Check sheet for the modelled part. Datum: model origin and axes. Units: mm. Round coordinates to 2 decimals unless told otherwise and drop trailing zeros. Order: outer loops, then holes, each group sorted by start corner. A loop starts at its lowest first (then second) coordinate and runs counter-clockwise, first axis right, second up. Notation, with made-up numbers: (87, 1) -> (108, 1) arc R14 ccw to (108, 27) -> close; hole circle Ø6 at (-30, 72.25). An arc over 180 degrees is marked (long way). Answer in a Markdown table with one row per item.
```python
from build123d import *

# Parameters (mm, degrees)
BOSS_EXTRUDE1_DEPTH = 250
BOSS_EXTRUDE3_START = -17.1
SKETCH3_W           = 10
SKETCH3_H           = 10
SKETCH3_R           = 1.75
BOSS_EXTRUDE3_DEPTH = 7
FILLET1_R           = 5
SKETCH5_R           = 1.5
CUT_EXTRUDE1_DEPTH  = 7
SKETCH6_W           = 20
SKETCH6_H           = 5
BOSS_EXTRUDE4_DEPTH = 7
SKETCH2_R           = 8.1
BOSS_EXTRUDE5_DEPTH = 5
BOSS_EXTRUDE6_START = -25
SKETCH2_3_R         = 8.1
BOSS_EXTRUDE6_DEPTH = 5
SKETCH7_R           = 1.5
CUT_EXTRUDE2_DEPTH  = 254.574446662


with BuildPart() as part:
    # Sketch1 → Boss-Extrude1 (new body)
    with BuildSketch(Plane.XY):
        Polygon((25, 20), (30, 20), (30, 0), (0, 0), (0, 20), (5, 20), (5, 5), (25, 5), align=None)
    extrude(amount=BOSS_EXTRUDE1_DEPTH)

    # Sketch3 → Boss-Extrude3 (add)
    with BuildSketch(Plane(origin=(30, 0, 0), x_dir=(0, 0, -1), z_dir=(1, 0, 0)).offset(BOSS_EXTRUDE3_START)):
        with Locations((-220, -5)):
            Rectangle(SKETCH3_W, SKETCH3_H)
        with Locations(Location((-220, -5, 0), (0, 0, 90))):
            Circle(SKETCH3_R, mode=Mode.SUBTRACT)
    extrude(amount=BOSS_EXTRUDE3_DEPTH)

    # Fillet1
    fillet1_edges = [part.edges().sort_by_distance(p)[0] for p in [
        (16.4, -10, 215),
        (16.4, -10, 225),
    ]]
    fillet(fillet1_edges, radius=FILLET1_R - 0.0001)  # a hair under: the kernel refuses the full size

    # Sketch5 → Cut-Extrude1 (cut)
    with BuildSketch(Plane(origin=(0, 5, 0), x_dir=(1, 0, 0), z_dir=(0, 1, 0))):
        with Locations(Location((15, -230, 0), (0, 0, 270))):
            Circle(SKETCH5_R)
        with Locations(Location((15, -210, 0), (0, 0, 270))):
            Circle(SKETCH5_R)
        with Locations(Location((15, -40, 0), (0, 0, 270))):
            Circle(SKETCH5_R)
        with Locations(Location((15, -20, 0), (0, 0, 270))):
            Circle(SKETCH5_R)
    extrude(amount=-CUT_EXTRUDE1_DEPTH, mode=Mode.SUBTRACT)

    # Sketch6 → Boss-Extrude4 (add)
    with BuildSketch(Plane(origin=(0, 20, 0), x_dir=(1, 0, 0), z_dir=(0, 1, 0))):
        with Locations((15, -2.5)):
            Rectangle(SKETCH6_W, SKETCH6_H)
        with Locations((15, -247.5)):
            Rectangle(SKETCH6_W, SKETCH6_H)
    extrude(amount=-BOSS_EXTRUDE4_DEPTH)

    # Sketch2 → Boss-Extrude5 (add)
    with BuildSketch(Plane(origin=(30, 0, 0), x_dir=(0, 0, -1), z_dir=(1, 0, 0))):
        with BuildLine():
            Line((-140, -15), (-140, -10))
            ThreePointArc((-140, -10), (-142.928932188, -2.928932188), (-150, 0))
            Line((-150, 0), (-100, 0))
            ThreePointArc((-100, 0), (-107.071067812, -2.928932188), (-110, -10))
            Line((-110, -10), (-110, -15))
            ThreePointArc((-110, -15), (-125, -30), (-140, -15))
        make_face()
        with Locations(Location((-125, -15, 0), (0, 0, 90))):
            Circle(SKETCH2_R, mode=Mode.SUBTRACT)
    extrude(amount=-BOSS_EXTRUDE5_DEPTH)

    # Sketch2<3> → Boss-Extrude6 (add)
    with BuildSketch(Plane(origin=(30, 0, 0), x_dir=(0, 0, -1), z_dir=(1, 0, 0)).offset(BOSS_EXTRUDE6_START)):
        with BuildLine():
            Line((-140, -15), (-140, -10))
            ThreePointArc((-140, -10), (-142.928932188, -2.928932188), (-150, 0))
            Line((-150, 0), (-100, 0))
            ThreePointArc((-100, 0), (-107.071067812, -2.928932188), (-110, -10))
            Line((-110, -10), (-110, -15))
            ThreePointArc((-110, -15), (-125, -30), (-140, -15))
        make_face()
        with Locations(Location((-125, -15, 0), (0, 0, 90))):
            Circle(SKETCH2_3_R, mode=Mode.SUBTRACT)
    extrude(amount=-BOSS_EXTRUDE6_DEPTH)

    # Sketch7 → Cut-Extrude2 (cut, through all)
    with BuildSketch(Plane.ZY):
        with Locations((115, 2)):
            Circle(SKETCH7_R)
        with Locations((135, 2)):
            Circle(SKETCH7_R)
    extrude(amount=-CUT_EXTRUDE2_DEPTH, mode=Mode.SUBTRACT)


solid = part.part
```
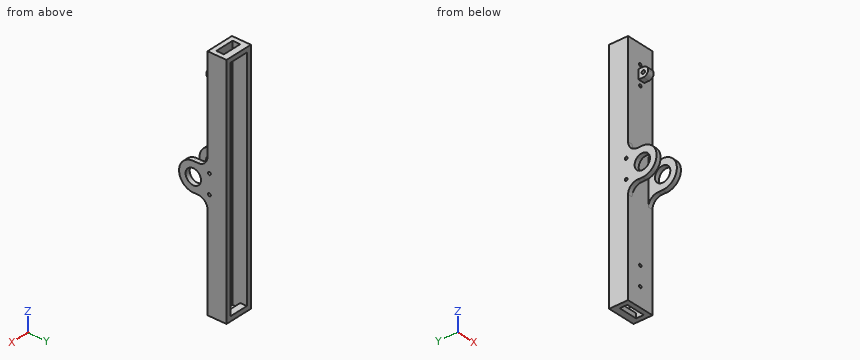
(1) Scan lines: probe 1 along Z at (x, y) = (18, -5); probe 2 along X at (y, z) = (6, 59); probe 3 along Y at (x, z) = (17.5, 220). Record each from-to range of solid material in increasing order. Write a range as from..to.
Solutions:
| item | result |
|---|---|
| probe 1 | 215..218.25, 221.75..225 |
| probe 2 | 0..5, 25..30 |
| probe 3 | -10..-6.75, -3.25..5 |
(2) Section check A-A on z = 81. Record the boundary of the cut face in (x, y).
Solutions:
| item | result |
|---|---|
| outline | (0, 0) -> (30, 0) -> (30, 20) -> (25, 20) -> (25, 5) -> (5, 5) -> (5, 20) -> (0, 20) -> close |
(3) Depth check by flat-ended pin: pin 1 Ø3.5 at (y, z) = (2, 115) entering from +X; pin 2 Ø5 at (x, y) = (24.5, -6.5) entering from +Z; pin 3 Ø1.5 at (x, z) = (18.5, 246.5) entering from -Y; pin 4 Ø10 at (x, z) = (20.5, 215.5) entering from -Y. Enter the tip coordinate at first touch or a pass-through.
Solutions:
| item | result |
|---|---|
| pin 1 | x = 30 |
| pin 2 | z = 141.96 |
| pin 3 | y = 0 |
| pin 4 | y = -10 |
(4) Section check B-B on y = -26. Record the boundary of the cut face in (x, z), plus the area to 3 significant figures.
Solutions:
| item | result |
|---|---|
| outline | (0, 114.8) -> (5, 114.8) -> (5, 135.2) -> (0, 135.2) -> close; (25, 114.8) -> (30, 114.8) -> (30, 135.2) -> (25, 135.2) -> close |
| area | 204 mm^2 |
